from build123d import *

# Parameters (mm, degrees)
SKETCH1_W           = 68.58
SKETCH1_H           = 53.26
SKETCH1_R           = 1.63195
BOSS_EXTRUDE1_DEPTH = 1.56
SKETCH2_W           = 16
SKETCH2_H           = 12
BOSS_EXTRUDE2_DEPTH = 11


with BuildPart() as part:
    # Sketch1 → Boss-Extrude1 (new body)
    with BuildSketch(Plane(origin=(0, 0, 0), x_dir=(1, 0, 0), z_dir=(0, 1, 0))):
        with Locations((31.75, 19.01)):
            Rectangle(SKETCH1_W, SKETCH1_H)
        Circle(SKETCH1_R, mode=Mode.SUBTRACT)
        with Locations((0, 27.9)):
            Circle(SKETCH1_R, mode=Mode.SUBTRACT)
        with Locations((51.9, -4.7)):
            Circle(SKETCH1_R, mode=Mode.SUBTRACT)
        with Locations((50.6, 43.1)):
            Circle(SKETCH1_R, mode=Mode.SUBTRACT)
    extrude(amount=BOSS_EXTRUDE1_DEPTH)

    # Sketch2 → Boss-Extrude2 (add)
    with BuildSketch(Plane(origin=(0, 0, 0), x_dir=(-1, 0, 0), z_dir=(0, -1, 0))):
        with Locations((-64.54, 30.64)):
            Rectangle(SKETCH2_W, SKETCH2_H)
    extrude(amount=BOSS_EXTRUDE2_DEPTH)


solid = part.part
The model under review builds one solid part; all positions refer to its coordinate system, in mm. A direction names the side the tool comes from. Round coordinates to 2 decimals unless told otherwise and drop trailing zeros. Write each loop counter-clockwise with the first axis right and the second up, starting at its lowest first coordinate (ties: lowest second). Pieces come first, ordered by that corner, then holes. Notation, with made-up numbers: M -33,51.5 L 10,51.5 A17 ccw 10,60.5 Z; hole C -9.5,44.5 d6. An arc over 180 degrees is marked long. Use a Markdown table: item, result. Add a question column.
Q1. We need section C-C, the plane z = -35. State the section outline as (x, y) points.
Q2. Insertion check: pin 1 (5.5 mm diameter, centred on y = -6.5, z = -31, fed in from -X); pin 2 (1.2 mm diameter, centred on y = 1, z = -10.5, fed in from +X); pin 3 (5 mm diameter, centred on x = 51.9, z = 4.7, fed in from -Y). Each pin has a flat end and moves straight along its axis. Give the tip position at first contact, or say it passes through.
Q3. We need section D-D, the plane x = 24.5. State the section outline as (y, z) points.
Q4. Machinability: for faces 1 (the face through (65, -5, -24.64)), 2 (the face through (66.04, 1, -19)), 3 (the face through (65, -5, -36.64)), 4 (the face through (31, 1.56, -19)), which of the approach directions +Z, -Z, +X, -X, +Y, -Y give a long, thin tool a straight path to every point of the face, cutting with its end or side? Answer none if there is none.
Q5. To check wall thickness, follow line 1 (Z direction, x = 0, y = 0.8); line 2 (X direction, y = 0.6, z = -43.1); line 3 (Z direction, x = 51.9, y = 0.5). State the ranges of each line that lie inside material, in increasing order.
Q6. We need section A-A, the plane x = 0. State the section outline as (y, z) points, plus the area to 3 significant figures.
Q7. We need section B-B, the plane z = 4.7. State the section outline as (x, y) points, plus the area to 3 significant figures.
Q8. The part is to be moulded in two halves that separate along X. For faces 5 (the face through (-0.354, 0.769, -26.307)), 6 (the face through (31, 1, -45.64)), 7 (the face through (56.54, -5, -31)), say which applies: pulls with the +X half, pulls with the -X half, needs draft (parallel to the pull), parting line crosses it, or undercut.
Findings below:
| question | item | result |
|---|---|---|
| 1 | outline | M -2.54,0 L 56.54,0 L 56.54,-11 L 72.54,-11 L 72.54,0 L 66.04,0 L 66.04,1.56 L -2.54,1.56 Z |
| 2 | pin 1 | stops at x = 56.54 |
| 2 | pin 2 | stops at x = 66.04 |
| 2 | pin 3 | stops at y = 0 |
| 3 | outline | M 0,-45.64 L 1.56,-45.64 L 1.56,7.62 L 0,7.62 Z |
| 4 | face 1 | +Z, +X, -X, -Y |
| 4 | face 2 | +Z, -Z, +X, +Y |
| 4 | face 3 | -Z, +X, -X, -Y |
| 4 | face 4 | +Z, -Z, +X, -X, +Y |
| 5 | line 1 | z = -45.64 to -29.53, -26.27 to -1.63, 1.63 to 7.62 |
| 5 | line 2 | x = -2.54 to 48.97, 52.23 to 66.04 |
| 5 | line 3 | z = -45.64 to -44.09, -42.11 to 3.07, 6.33 to 7.62 |
| 6 | outline | M 0,-45.64 L 1.56,-45.64 L 1.56,-29.53 L 0,-29.53 Z; M 0,-26.27 L 1.56,-26.27 L 1.56,-1.63 L 0,-1.63 Z; M 0,1.63 L 1.56,1.63 L 1.56,7.62 L 0,7.62 Z |
| 6 | area | 72.9 mm² |
| 7 | outline | M -2.54,0 L 50.27,0 L 50.27,1.56 L -2.54,1.56 Z; M 53.53,0 L 66.04,0 L 66.04,1.56 L 53.53,1.56 Z |
| 7 | area | 102 mm² |
| 8 | face 5 | undercut |
| 8 | face 6 | needs draft |
| 8 | face 7 | pulls with the -X half |
